Design review of the part built by this model. Coordinates are the model's own, in mm. A direction names the side the tool comes from. Round coordinates to 2 decimals unless told otherwise and drop trailing zeros. Order: outer loops, then holes, each group sorted by start corner. A loop starts at its lowest first (then second) coordinate and runs counter-clockwise, first axis right, second up. Notation, with made-up numbers: (69, 24.25) - (109, 24.25) arc R7 cw to (109, 36.25) - close; hole circle Ø10 at (81.25, 84). An arc over 180 degrees is marked (long way). Write item = value, one per line.
from build123d import *

# Parameters (mm, degrees)
F0_R     = 7
F0_R_2   = 5.5
F1_DEPTH = 44
F2_DEPTH = 19
F5_DEPTH = 24
F6_DEPTH = 19


with BuildPart() as f1:
    # F0 (on Front) → F1 (new body)
    with BuildSketch(Plane.XZ):
        Polygon((-14, 11), (-14, -7), (-7, -14), (20, -14), (20, 14.4734603858), (0, 18), (-7, 18), align=None)
        Circle(F0_R, mode=Mode.SUBTRACT)
        with BuildLine():
            Line((20, 14.4734603858), (20, -14))
            Line((20, -14), (25.5755389113, -14))
            Line((25.5755389113, -14), (59.2058823529, -14))
            Line((59.2058823529, -14), (72, 1))
            Line((72, 1), (72, 20))
            Line((72, 20), (67, 25))
            Line((67, 25), (43, 25))
            ThreePointArc((43, 25), (34.5610987057, 15.9820441422), (22.3613808358, 14.0570852328))
            Line((22.3613808358, 14.0570852328), (20, 14.4734603858))
        make_face()
        with Locations((58, 11)):
            Circle(F0_R_2, mode=Mode.SUBTRACT)
        with BuildLine():
            Line((59.2058823529, -14), (25.5755389113, -14))
            ThreePointArc((25.5755389113, -14), (28.8407746924, -15.2134137678), (30.5211776528, -18.2647058824))
            ThreePointArc((30.5211776528, -18.2647058824), (32.8580078559, -26.115672061), (37.2969800527, -33))
            Line((37.2969800527, -33), (43, -33))
            Line((43, -33), (59.2058823529, -14))
        make_face()
    extrude(amount=-F1_DEPTH)

    # F0 (on Front) → F2 (cut)
    with BuildSketch(Plane.XZ):
        Polygon((-14, 11), (-14, -7), (-7, -14), (20, -14), (20, 14.4734603858), (0, 18), (-7, 18), align=None)
        Circle(F0_R, mode=Mode.SUBTRACT)
    extrude(amount=-F2_DEPTH, mode=Mode.SUBTRACT)

    # F4 (on offset) → F5 (cut)
    with BuildSketch(Plane(origin=(0, 32, 0), x_dir=(-1, 0, 0), z_dir=(0, 1, 0))):
        with BuildLine():
            Line((-79.095418143, 42.8479425609), (-79.095418143, -13.075442161))
            ThreePointArc((-79.095418143, -13.075442161), (-39.789926782, 1.9384056037), (-34.4063231516, 43.6679405614))
            Line((-34.4063231516, 43.6679405614), (-79.095418143, 42.8479425609))
        make_face()
    extrude(amount=-F5_DEPTH, mode=Mode.SUBTRACT)

    # F0 (on Front) → F6 (cut)
    with BuildSketch(Plane.XZ):
        with BuildLine():
            Line((59.2058823529, -14), (25.5755389113, -14))
            ThreePointArc((25.5755389113, -14), (28.8407746924, -15.2134137678), (30.5211776528, -18.2647058824))
            ThreePointArc((30.5211776528, -18.2647058824), (32.8580078559, -26.115672061), (37.2969800527, -33))
            Line((37.2969800527, -33), (43, -33))
            Line((43, -33), (59.2058823529, -14))
        make_face()
    extrude(amount=-F6_DEPTH, mode=Mode.SUBTRACT)


solid = f1.part
Item 1: The part is to be moulded in two halves that separate along X. For faces 4 (the face through (6.466, 31.325, -2.681)), 5 (the face through (53, 32, 7)), 6 (the face through (70, 4, 22)), 7 (the face through (-14, 31, 2)), say which applies: +X half, -X half, draft (parallel to the pull), parting line (faces both ways), or undercut.
Data:
face_4 = undercut
face_5 = draft
face_6 = +X half
face_7 = -X half
Item 2: For faces 1 (the face through (20, 9, 0)), 2 (the face through (-3, 31, 18)), 3 (the face through (42, 19, -21)), list the 3-axis set-ups (+Z, -Z, +X, -X, +Y, -Y) from which the entire face can be reached by the end or side of a thin tool; tool diameter is ignored.
Data:
face_1 = +Z, -Z, -X, -Y
face_2 = +Z, -X, +Y, -Y
face_3 = -Z, +X, -X, -Y
Item 3: Take a section at D-D, the plane y = 14. State the section outline as (x, z) points.
Data:
outline = (20, -14) - (59.21, -14) - (60.8, -12.13) arc R41 cw to (32.84, 15.18) arc R19 cw to (22.36, 14.06) - (20, 14.47) - close
Item 4: Insertion check: P1, Ø16, axis at x = 8.5, z = 0, coming from the -Y side; P2, Ø5, axis at y = 6.5, z = 16, coming from the -X side; P3, Ø5, axis at x = 17, y = 13.5, coming from the -Z side; P4, Ø7.5, axis at x = -4, y = 32.5, coming from the +Z side. Each pin has a flat end and moves straight along its axis. Give the tip position at first contact, or say it passes through.
Data:
P1 = 19
P2 = 20
P3 = through
P4 = 18
Item 5: Take a section at B-B, the plane z = 0. State the section outline as (x, y) points, and give its area (3 significant figures).
Data:
outline = (-14, 19) - (-7, 19) - (-7, 44) - (-14, 44) - close; (7, 19) - (20, 19) - (20, 0) - (71.15, 0) - (71.15, 8) - (41.42, 8) - (41.42, 32) - (71.15, 32) - (71.15, 44) - (7, 44) - close
area = 2,040 mm2
Item 6: For line 1 along Z through (x, y) = (0, 32.75); line 2 along Y through (x, z) = (57, 1.5); line 3 along Z through (x, y) = (58, 6.25), list the stretches that pass through material, from the lowest coordinate up. Write a range as [from, to].
Data:
line_1 = [-14, -7], [7, 18]
line_2 = [0, 8], [32, 44]
line_3 = [-14, 5.5], [16.5, 25]
Item 7: Take a section at A-A, the plane y = 30. State the section outline as (x, z) points, and give its area (3 significant figures).
Data:
outline = (-14, -7) - (-7, -14) - (25.58, -14) arc R5 cw to (30.52, -18.26) arc R29 ccw to (37.3, -33) - (43, -33) - (60.8, -12.13) arc R41 cw to (32.84, 15.18) arc R19 cw to (22.36, 14.06) - (0, 18) - (-7, 18) - (-14, 11) - close; hole circle Ø14 at (0, 0)
area = 1,870 mm2
Item 8: Take a section at C-C, the plane x = 66. State the section outline as (y, z) points.
Data:
outline = (0, -6.03) - (8, -6.03) - (8, 25) - (0, 25) - close; (32, -6.03) - (44, -6.03) - (44, 25) - (32, 25) - close
